from build123d import *

# Parameters (mm, degrees)
SKIZZE1_R                       = 2
SKIZZE1_R_2                     = 1.45
AUFSATZ_LINEAR_AUSTRAGEN1_DEPTH = 6
SKIZZE2_R                       = 2.15
SKIZZE2_R_2                     = 1.755690243
AUFSATZ_LINEAR_AUSTRAGEN2_DEPTH = 1.8
AUFSATZ_LINEAR_START            = -2.6
SKIZZE2_2_R                     = 2.15
SKIZZE2_2_R_2                   = 1.755690243
AUFSATZ_LINEAR_AUSTRAGEN3_DEPTH = 1.9
FASE1_SIZE                      = 0.15
FASE2_SIZE                      = 0.15


with BuildPart() as part:
    # Skizze1 → Aufsatz-Linear austragen1 (new body)
    with BuildSketch(Plane.XY):
        Circle(SKIZZE1_R)
        Circle(SKIZZE1_R_2, mode=Mode.SUBTRACT)
    extrude(amount=AUFSATZ_LINEAR_AUSTRAGEN1_DEPTH)

    # Skizze2 → Aufsatz-Linear austragen2 (add)
    with BuildSketch(Plane(origin=(0, 0, 0), x_dir=(-1, 0, 0), z_dir=(0, 0, -1))):
        Circle(SKIZZE2_R)
        Circle(SKIZZE2_R_2, mode=Mode.SUBTRACT)
    extrude(amount=-AUFSATZ_LINEAR_AUSTRAGEN2_DEPTH)

    # Skizze2<2> → Aufsatz-Linear austragen3 (add)
    with BuildSketch(Plane(origin=(0, 0, 0), x_dir=(-1, 0, 0), z_dir=(0, 0, -1)).offset(AUFSATZ_LINEAR_START)):
        Circle(SKIZZE2_2_R)
        Circle(SKIZZE2_2_R_2, mode=Mode.SUBTRACT)
    extrude(amount=-AUFSATZ_LINEAR_AUSTRAGEN3_DEPTH)

    # Fase1
    fase1_edges = [part.edges().sort_by_distance(p)[0] for p in [
        (2.15, 0, 0),
        (-2, 0, 6),
        (-1.45, 0, 0),
        (-1.45, 0, 6),
    ]]
    chamfer(fase1_edges, length=FASE1_SIZE)

    # Fase2
    fase2_edges = [part.edges().sort_by_distance(p)[0] for p in [
        (2.15, 0, 1.8),
        (2.15, 0, 4.5),
        (2.15, 0, 2.6),
    ]]
    chamfer(fase2_edges, length=FASE2_SIZE - 0.0001)  # a hair under: the kernel refuses the full size


solid = part.part
Read the model definition and answer for the solid it produces. Units are mm, in the model's axes. A direction names the side the tool comes from. Give positions to 0.01 mm unless a question says otherwise; leave off trailing zeros. Write each loop counter-clockwise with the first axis right and the second up, starting at its lowest first coordinate (ties: lowest second). Pieces come first, ordered by that corner, then holes. Notation, with made-up numbers: (6.25, -31) - (43.25, -31) arc R17 cw to (43.25, -14) - close; hole circle Ø10 at (-24, 16.25). An arc over 180 degrees is marked (long way). Answer in a Markdown table with one row per item. Add a question column.
Item 1: Find the intervals of material crossed by L1, parallel to Y at x = 0, z = 2.35; L2, parallel to Y at x = 0, z = 3.7; L3, parallel to Z at x = 2, y = -0.45, in increasing order.
Item 2: Flat-ended cylindrical pins translate along their axes: P1, Ø1.5, axis at x = 1, z = 1, coming from the +Y side; P2, Ø2.5, axis at x = 0, y = 0, coming from the -Z side. Find the tip coordinate at first contact, or state that the pin passes through.
Item 3: Determine the mould class of faces 4 (the face through (2.15, 0.09, 0.89)), 5 (the face through (-1.45, 0.06, 2.96)) for opening direction Y: pulls with the +Y half, pulls with the -Y half, needs draft (parallel to the pull), parting line crosses it, or undercut.
Item 4: Section C-C, the plane z = 2.5 is taken. Write down the section's boundary in (x, y).
Item 5: Section D-D, the plane z = 4.25 is taken. Write down the section's boundary in (x, y), and give its area (3 significant figures).
Item 6: A tool of negligible diameter and unlimited length cuts with its end or side. For faces 1 (the face through (0, -2, 2)), 2 (the face through (0, -2, 5)), 3 (the face through (2.15, 0.09, 3.54)), from which of +Z, -Z, +X, -X, +Y, -Y can it reach the whole face along a straight path? Write none if from no direction.
Recorded:
| question | item | result |
|---|---|---|
| 1 | L1 | y = -2 to -1.45, 1.45 to 2 |
| 1 | L2 | y = -2.15 to -1.45, 1.45 to 2.15 |
| 1 | L3 | z = 0.05 to 1.75, 2.65 to 4.45 |
| 2 | P1 | stops at y = 2.14 |
| 2 | P2 | passes through |
| 3 | face 4 | parting line crosses it |
| 3 | face 5 | undercut |
| 4 | outline | circle Ø4 at (0, 0); hole circle Ø2.9 at (0, 0) |
| 5 | outline | circle Ø4.3 at (0, 0); hole circle Ø2.9 at (0, 0) |
| 5 | area | 7.92 mm2 |
| 6 | face 1 | none |
| 6 | face 2 | +Z |
| 6 | face 3 | +Z, -Z |
